from build123d import *

# Parameters (mm, degrees)
SKETCH1_W           = 50
SKETCH1_H           = 38.5
SKETCH1_R           = 8
BOSS_EXTRUDE1_DEPTH = 22
CUT_EXTRUDE5_DEPTH  = 45
SKETCH2_R           = 2.15
CUT_EXTRUDE1_DEPTH  = 39.5
SKETCH3_R           = 2.5
CUT_EXTRUDE2_DEPTH  = 12
SKETCH4_R           = 14
CUT_EXTRUDE3_DEPTH  = 1
SKETCH5_R           = 14
CUT_EXTRUDE4_DEPTH  = 1


with BuildPart() as part:
    # Sketch1 → Boss-Extrude1 (new body, symmetric)
    with BuildSketch(Plane.XY):
        Rectangle(SKETCH1_W, SKETCH1_H)
        with Locations((0, 0.25)):
            Circle(SKETCH1_R, mode=Mode.SUBTRACT)
    extrude(amount=BOSS_EXTRUDE1_DEPTH, both=True)

    # Sketch6 → Cut-Extrude5 (cut, through all)
    with BuildSketch(Plane.XY.offset(22)):
        Polygon((-25, -13.25), (-12, -13.25), (-6.965402213, -19.25), (-25, -19.25), align=None)
        Polygon((25, -13.25), (12, -13.25), (6, -19.25), (25, -19.25), align=None)
    extrude(amount=-CUT_EXTRUDE5_DEPTH, mode=Mode.SUBTRACT)

    # Sketch2 → Cut-Extrude1 (cut, through all)
    with BuildSketch(Plane(origin=(0, 19.25, 0), x_dir=(-1, 0, 0), z_dir=(0, -1, 0))):
        with Locations((18, -17)):
            Circle(SKETCH2_R)
        with Locations((-18, -17)):
            Circle(SKETCH2_R)
        with Locations((-18, 17)):
            Circle(SKETCH2_R)
        with Locations((18, 17)):
            Circle(SKETCH2_R)
    extrude(amount=CUT_EXTRUDE1_DEPTH, mode=Mode.SUBTRACT)

    # Sketch3 → Cut-Extrude2 (cut)
    with BuildSketch(Plane.XZ.offset(-19.25)):
        with Locations((-18, 17)):
            Circle(SKETCH3_R)
        with Locations((18, 17)):
            Circle(SKETCH3_R)
        with Locations((18, -17)):
            Circle(SKETCH3_R)
        with Locations((-18, -17)):
            Circle(SKETCH3_R)
    extrude(amount=CUT_EXTRUDE2_DEPTH, mode=Mode.SUBTRACT)

    # Sketch4 → Cut-Extrude3 (cut)
    with BuildSketch(Plane.XY.offset(22)):
        with Locations((0, 0.25)):
            Circle(SKETCH4_R)
    extrude(amount=-CUT_EXTRUDE3_DEPTH, mode=Mode.SUBTRACT)

    # Sketch5 → Cut-Extrude4 (cut)
    with BuildSketch(Plane(origin=(0, 0, -22), x_dir=(-1, 0, 0), z_dir=(0, 0, -1))):
        with Locations((0, 0.25)):
            Circle(SKETCH5_R)
    extrude(amount=-CUT_EXTRUDE4_DEPTH, mode=Mode.SUBTRACT)


solid = part.part
The listing builds one solid part. Answer for the finished solid, in the listing's coordinates (mm). A direction names the side the tool comes from. Round coordinates to 2 decimals unless told otherwise and drop trailing zeros. Write each loop counter-clockwise with the first axis right and the second up, starting at its lowest first coordinate (ties: lowest second). Pieces come first, ordered by that corner, then holes. Notation, with made-up numbers: (64.5, 13.5) - (82.5, 13.5) arc R23 cw to (82.5, 44.5) - close; hole circle Ø6 at (7, 28.5). An arc over 180 degrees is marked (long way). Use a Markdown table: item, result. Add a question column.
1. For a pull along Z with two mould halves and no side action, classify faces 5 (the face through (-20.5, 13.3, 17.1)), 6 (the face through (6, -6, 21)), 7 (the face through (-19, -13.25, 0)) as +Z half, -Z half, draft (parallel to the pull), parting line (faces both ways), or undercut.
2. The part is cut by section D-D (x = 0). Write down the section's boundary in (y, z).
3. A tool of negligible diameter and unlimited length cuts with its end or side. For faces 1 (the face through (-11.5, 8.8, 22)), 2 (the face through (19, -13.25, 0)), 3 (the face through (-12.932, -5.112, -21.507)), 4 (the face through (-20.5, 13.3, -16.9)), from which of +Z, -Z, +X, -X, +Y, -Y can it reach the whole face along a straight path? Write none if from no direction.
4. A flat-ended cylindrical pin translates along its axis: P1, Ø6.5, axis at x = 20, z = -6, coming from the -Y side. Find the tip coordinate at first contact, or state that the pin passes through.
5. Consider line 1 (Z direction, x = -18, y = -6); line 2 (Z direction, x = 18, y = 11.75); line 3 (X direction, y = 16.5, z = 19). Determine where each line is inside the solid, lowest interval first.
6. The part is cut by section C-C (z = -12). Write down the section's boundary in (x, y).
7. The part is cut by section A-A (z = 17). Write down the section's boundary in (x, y), and give its area (3 significant figures).
8. The part is cut by section B-B (x = 18). Write down the section's boundary in (y, z).
Reported:
| question | item | result |
|---|---|---|
| 1 | face 5 | undercut |
| 1 | face 6 | +Z half |
| 1 | face 7 | draft |
| 2 | outline | (-19.25, -22) - (-13.75, -22) - (-13.75, -21) - (-7.75, -21) - (-7.75, 21) - (-13.75, 21) - (-13.75, 22) - (-19.25, 22) - close; (8.25, -21) - (14.25, -21) - (14.25, -22) - (19.25, -22) - (19.25, 22) - (14.25, 22) - (14.25, 21) - (8.25, 21) - close |
| 3 | face 1 | +Z, +X, -X, +Y, -Y |
| 3 | face 2 | +Z, -Z, +X, -Y |
| 3 | face 3 | -Z |
| 3 | face 4 | +Y |
| 4 | P1 | y = -13.25 |
| 5 | line 1 | -22 to -19.15, -14.85 to 14.85, 19.15 to 22 |
| 5 | line 2 | -22 to -19.5, -14.5 to 14.5, 19.5 to 22 |
| 5 | line 3 | -25 to -19.5, -16.5 to 16.5, 19.5 to 25 |
| 6 | outline | (-25, -13.25) - (-12, -13.25) - (-6.97, -19.25) - (6, -19.25) - (12, -13.25) - (25, -13.25) - (25, 19.25) - (-25, 19.25) - close; hole circle Ø16 at (0, 0.25) |
| 7 | outline | (-25, -13.25) - (-20.15, -13.25) - (-20.15, 7.25) - (-20.5, 7.25) - (-20.5, 19.25) - (-25, 19.25) - close; (-15.85, -13.25) - (-12, -13.25) - (-6.97, -19.25) - (6, -19.25) - (12, -13.25) - (15.85, -13.25) - (15.85, 7.25) - (15.5, 7.25) - (15.5, 19.25) - (-15.5, 19.25) - (-15.5, 7.25) - (-15.85, 7.25) - close; (20.15, -13.25) - (25, -13.25) - (25, 19.25) - (20.5, 19.25) - (20.5, 7.25) - (20.15, 7.25) - close; hole circle Ø16 at (0, 0.25) |
| 7 | area | 1,240 mm^2 |
| 8 | outline | (-13.25, -22) - (19.25, -22) - (19.25, -19.5) - (7.25, -19.5) - (7.25, -19.15) - (-13.25, -19.15) - close; (-13.25, -14.85) - (7.25, -14.85) - (7.25, -14.5) - (19.25, -14.5) - (19.25, 14.5) - (7.25, 14.5) - (7.25, 14.85) - (-13.25, 14.85) - close; (-13.25, 19.15) - (7.25, 19.15) - (7.25, 19.5) - (19.25, 19.5) - (19.25, 22) - (-13.25, 22) - close |
